from build123d import *

# Parameters (mm, degrees)
ESBO_O1_R                = 12.2
RESSALTO_EXTRUS_O1_DEPTH = 30.8
FILETE1_R                = 1
ESBO_O2_R                = 2
RESSALTO_EXTRUS_O2_DEPTH = 10
ESBO_O4_W                = 0.958903526
ESBO_O4_H                = 3.564219336
ESBO_O4_W_2              = 0.894406544
RESSALTO_EXTRUS_O3_DEPTH = 5
FILETE2_R                = 1
ESBO_O5_R                = 0.782109668
CORTE_EXTRUS_O2_DEPTH    = 48.924150269


with BuildPart() as part:
    # Esboço1 → Ressalto-extrusão1 (new body)
    with BuildSketch(Plane.XY):
        with Locations(Location((0, 0, 0), (0, 0, 180))):
            Circle(ESBO_O1_R)
    extrude(amount=RESSALTO_EXTRUS_O1_DEPTH)

    # Filete1
    filete1_edges = [part.edges().sort_by_distance(p)[0] for p in [
        (12.2, 0, 0),
        (12.2, 0, 30.8),
    ]]
    fillet(filete1_edges, radius=FILETE1_R)

    # Esboço2 → Ressalto-extrusão2 (add)
    with BuildSketch(Plane.XY.offset(30.8)):
        Circle(ESBO_O2_R)
    extrude(amount=RESSALTO_EXTRUS_O2_DEPTH)

    # Esboço4 → Ressalto-extrusão3 (add)
    with BuildSketch(Plane(origin=(0, 0, 0), x_dir=(-1, 0, 0), z_dir=(0, 0, -1))):
        with Locations((-9.303363775, 0.548104497)):
            Rectangle(ESBO_O4_W, ESBO_O4_H)
        with Locations((8.369776419, 0.548104497)):
            Rectangle(ESBO_O4_W_2, ESBO_O4_H)
    extrude(amount=RESSALTO_EXTRUS_O3_DEPTH)

    # Filete2
    filete2_edges = [part.edges().sort_by_distance(p)[0] for p in [
        (9.303363775, -1.234005171, -5),
        (9.303363775, 2.330214165, -5),
        (-8.369776419, 2.330214165, -5),
        (-8.369776419, -1.234005171, -5),
    ]]
    fillet(filete2_edges, radius=FILETE2_R)

    # Esboço5 → Corte-extrusão2 (cut, through all)
    with BuildSketch(Plane(origin=(9.782815538, 0, 0), x_dir=(0, 0, -1), z_dir=(1, 0, 0))):
        with Locations((3.47716986, 0.548104497)):
            Circle(ESBO_O5_R)
    extrude(amount=-CORTE_EXTRUS_O2_DEPTH, mode=Mode.SUBTRACT)


solid = part.part
Design review of the part built by this model. Coordinates are the model's own, in mm. A direction names the side the tool comes from. Give positions to 0.01 mm unless a question says otherwise; leave off trailing zeros. Loops run counter-clockwise (first coordinate to the right, second up) from the corner with the lowest first, then second, coordinate; pieces in that order, holes last. Notation, with made-up numbers: (29, 88) -> (77, 88) arc R24 ccw to (77, 111) -> close; hole circle Ø4 at (-29, 59.5). An arc over 180 degrees is marked (long way). One line per question, with ' | ' between items. Start each with the question number.
(1) We need section A-A (x = 0). State the section outline as (y, z) points, and give its area (3 significant figures).
(2) For line 1 (Z direction, x = -2, y = -4.5); line 2 (Y direction, x = 0, z = 6); line 3 (Z direction, x = 5, y = 11), list the stretches that pass through material, from the lowest coordinate up.
(3) Insertion check: P1, Ø1.4, axis at y = 0.55, z = -3.48, coming from the -X side; P2, Ø6, axis at x = 5, y = -4, coming from the +Z side; P3, Ø10, axis at x = 3.5, z = 35, coming from the -Y side; P4, Ø10, axis at x = -5, z = 35.5, coming from the +Y side. Each pin has a flat end and moves straight along its axis. Give the tip position at first contact, or say it passes through.
(4) Draft analysis for pull direction Z (two halves, no side actions). For faces 6 (the face through (9.31, 0.783, -4.223)), 7 (the face through (9.3, -0.95, -4.7)), 8 (the face through (-8.4, 2.33, -2)), 9 (the face through (-8.364, 0.783, -4.223)), state which applies: +Z half, -Z half, draft (parallel to the pull), parting line (faces both ways), or undercut.
(5) We need section B-B (z = 20). State the section outline as (x, y) points, and give its area (3 significant figures).
(6) For faces 1 (the face through (-8.817, 1, -2)), 2 (the face through (8.824, 1, -2)), 3 (the face through (9.783, 1, -2)), 4 (the face through (9, -1.234, -2)), 5 (the face through (9, 2.33, -2)), list the 3-axis set-ups (+Z, -Z, +X, -X, +Y, -Y) from which the entire face can be reached by the end or side of a thin tool; tool diameter is ignored.
The answers:
1) outline: (-12.2, 1) arc R1 ccw to (-11.2, 0) -> (11.2, 0) arc R1 ccw to (12.2, 1) -> (12.2, 29.8) arc R1 ccw to (11.2, 30.8) -> (2, 30.8) -> (2, 40.8) -> (-2, 40.8) -> (-2, 30.8) -> (-11.2, 30.8) arc R1 ccw to (-12.2, 29.8) -> close | area: 791 mm^2
2) line 1: z = 0 to 30.8 | line 2: y = -12.2 to 12.2 | line 3: z = 0.53 to 30.27
3) P1: passes through | P2: stops at z = 30.8 | P3: stops at y = -11.94 | P4: stops at y = 11.1
4) face 6: undercut | face 7: -Z half | face 8: draft | face 9: undercut
5) outline: circle Ø24.4 at (0, 0) | area: 468 mm^2
6) face 1: -Z, -X, +Y, -Y | face 2: -Z, +Y, -Y | face 3: -Z, +X, +Y, -Y | face 4: -Z, +X, -X, -Y | face 5: -Z, +X, -X, +Y
